from build123d import *

# Parameters (mm, degrees)
F0_W     = 63.4695142508
F0_H     = 51.2949377298
F0_W_2   = 61
F0_H_2   = 49
F1_DEPTH = 180
F3_W     = 2.2321660072
F3_H     = 3.732714802
F3_W_2   = 14.8959429935
F3_H_2   = 39.1232501715
F3_W_3   = 3.5938005894
F3_H_3   = 1.2999996543
F3_W_4   = 1.4519924298
F4_DEPTH = 10


# Not quite as in the source:
# - a feature names something its author has since deleted; it is built from what else it names
# - the program builds the solid bodies; features that only make, move or delete a surface that nothing else refers to are left out


with BuildPart() as f1:
    # F0 (on Top) → F1 (new body)
    with BuildSketch(Plane.XY):
        Rectangle(F0_W, F0_H)
        Rectangle(F0_W_2, F0_H_2, mode=Mode.SUBTRACT)
    extrude(amount=-F1_DEPTH)

    # F3 (on Top) → F4 (join)
    with BuildSketch(Plane.XY):
        with Locations((-25.2534588799, 22.6865075529)):
            Rectangle(F3_W, F3_H)
        Polygon((-24.1373758763, 20.8201501518), (-26.3695418835, 20.8201501518), (-26.3695418835, 18.7030434608), (-26.3695418835, -19.5201504976), (-22.775741294, -19.5201504976), (-22.775741294, -20.8201501518), (21.0672114044, -20.8201501518), (21.0672114044, -19.5201504976), (10.0216064602, -19.5201504976), (10.0216064602, 19.603099674), (22.2738981247, 19.603099674), (22.2738981247, 20.8201501518), align=None)
        with Locations((-17.7230439149, 0.1456094906)):
            Rectangle(F3_W_2, F3_H_2, mode=Mode.SUBTRACT)
        with Locations((0.6728977896, 0.226427801)):
            Rectangle(F3_W_2, F3_H_2, mode=Mode.SUBTRACT)
        Polygon((-26.3695418835, 18.7030434608), (-26.3695418835, 20.8201501518), (-26.3695418835, 24.5528649539), (-30.5465664715, 24.5528649539), (-30.5465664715, 18.7030434608), align=None)
        Polygon((22.2738981247, 24.4889948517), (22.2738981247, 20.8201501518), (26.3695418835, 20.8201501518), (26.3695418835, 19.603099674), (30.5195916444, 19.603099674), (30.5195916444, 24.4889948517), align=None)
        Polygon((26.3695418835, 20.8201501518), (22.2738981247, 20.8201501518), (22.2738981247, 19.603099674), (24.9175494537, 19.603099674), (26.3695418835, 19.603099674), align=None)
        with Locations((-24.5726415887, -20.1701503247)):
            Rectangle(F3_W_3, F3_H_3)
        Polygon((-26.3695418835, -20.8201501518), (-26.3695418835, -19.5201504976), (-30.8873578906, -19.5201504976), (-30.8873578906, -24.8510874808), (-22.775741294, -24.8510874808), (-22.775741294, -20.8201501518), align=None)
        with Locations((25.6435456686, 0.0414745882)):
            Rectangle(F3_W_4, F3_H_2)
        Polygon((31.1229377985, -19.5201504976), (26.3695418835, -19.5201504976), (26.3695418835, -20.8201501518), (21.0672114044, -20.8201501518), (21.0672114044, -24.8510874808), (31.1229377985, -24.8510874808), align=None)
        Polygon((26.3695418835, -20.8201501518), (26.3695418835, -19.5201504976), (24.9175494537, -19.5201504976), (21.0672114044, -19.5201504976), (21.0672114044, -20.8201501518), align=None)
    extrude(amount=-F4_DEPTH)


solid = f1.part
Work out the finished part from the listing and answer in its coordinate system (mm). A direction names the side the tool comes from. Coordinates: 2 decimals unless noted, no trailing zeros. Write each loop counter-clockwise with the first axis right and the second up, starting at its lowest first coordinate (ties: lowest second). Pieces come first, ordered by that corner, then holes. Notation, with made-up numbers: M 63,75.5 L 116,75.5 A21 cw 116,85.5 Z; hole C 26,-38.5 d2. An arc over 180 degrees is marked long. Use one line per item in the form item = value. Start each with the question number.
1. A tool of negligible diameter and unlimited length cuts with its end or side. For faces 4 (the face through (-30.5, 0, -89)), 5 (the face through (1, -19.335, -5)), from which of +Z, -Z, +X, -X, +Y, -Y can it reach the whole face along a straight path? Write none if from no direction.
2. This flat-tipped pin is pushed along its axis until it touches: P1, Ø6, axis at x = -14.5, y = 5, coming from the -Z side. Where does it stop, or does it pass through?
3. Straight lines are drawn through the part: probe 1 along Y at (x, z) = (-15, -166); probe 2 along X at (y, z) = (-17, -157.5); probe 3 along Z at (x, y) = (9, 11.5). For each, find the intervals that lie inside material, in ascending order. Write a range as from..to.
4. The part is cut by section C-C (z = -69). Give the vertices of the cut face in (x, y), plus the area to 3 significant figures.
5. The part is cut by section A-A (x = -2). Give the vertices of the cut face in (y, z), plus the area to 3 significant figures.
6. The part is cut by section B-B (y = -15). Give the vertices of the cut face in (x, z).
7. The mould has two halves that part along X. Classify faces 1 (the face through (-31, 0, -180)), 2 (the face through (-24.137, 23, -5)), 3 (the face through (-31.735, 0, -89)): released by +X, released by -X, zero draft, split by the parting line, or undercut.
Evaluation:
q1.face_4 = -Z
q1.face_5 = +Z, -Z
q2.P1 = through
q3.probe_1 = -25.65..-24.5, 24.5..25.65
q3.probe_2 = -31.73..-30.5, 30.5..31.73
q3.probe_3 = -10..0
q4.outline = M -31.73,-25.65 L 31.73,-25.65 L 31.73,25.65 L -31.73,25.65 Z; hole M -30.5,-24.5 L 30.5,-24.5 L 30.5,24.5 L -30.5,24.5 Z
q4.area = 267 mm^2
q5.outline = M -25.65,-180 L -24.5,-180 L -24.5,0 L -25.65,0 Z; M -20.82,-10 L -19.34,-10 L -19.34,0 L -20.82,0 Z; M 19.79,-10 L 20.82,-10 L 20.82,0 L 19.79,0 Z; M 24.5,-180 L 25.65,-180 L 25.65,0 L 24.5,0 Z
q5.area = 438 mm^2
q6.outline = M -31.73,-180 L -30.5,-180 L -30.5,0 L -31.73,0 Z; M -26.37,-10 L -25.17,-10 L -25.17,0 L -26.37,0 Z; M -10.28,-10 L -6.78,-10 L -6.78,0 L -10.28,0 Z; M 8.12,-10 L 10.02,-10 L 10.02,0 L 8.12,0 Z; M 24.92,-10 L 26.37,-10 L 26.37,0 L 24.92,0 Z; M 30.5,-180 L 31.73,-180 L 31.73,0 L 30.5,0 Z
q7.face_1 = zero draft
q7.face_2 = undercut
q7.face_3 = released by -X
